The listing builds one solid part. Answer for the finished solid, in the listing's coordinates (mm). Face numbers are marked on the shaded views. A direction names the side the tool comes from. Coordinates: 2 decimals unless noted, no trailing zeros. Order: outer loops, then holes, each group sorted by start corner. A loop starts at its lowest first (then second) coordinate and runs counter-clockwise, first axis right, second up. Notation, with made-up numbers: (23, -27.75) -> (68, -27.75) arc R13 ccw to (68, -5.75) -> close; hole circle Ø7 at (-28.5, -26). An arc over 180 degrees is marked (long way). Write item = value, one per line.
from build123d import *

# Parameters (mm, degrees)
SKETCH_1_W          = 133
SKETCH_1_H          = 140
EXTRUDE_1_DEPTH     = 140
SKETCH_2_W          = 113
SKETCH_2_H          = 100
CUT_EXTRUDE_1_DEPTH = 110
SKETCH_3_W          = 100
SKETCH_3_H          = 13
EXTRUDE_2_DEPTH     = 100
SKETCH_4_R          = 3
CUT_EXTRUDE_3_DEPTH = 217.846143613
SKETCH_5_W          = 12
SKETCH_5_H          = 12
EXTRUDE_3_DEPTH     = 10
SKETCH_6_R          = 14.490887282
SKETCH_6_R_2        = 4.490887282
EXTRUDE_2_2_DEPTH   = 12
SKETCH_7_R          = 4.490887282
CUT_EXTRUDE_4_DEPTH = 265.708919896


with BuildPart() as part:
    # 草圖1 → 填料-伸長1 (new body)
    with BuildSketch(Plane(origin=(0, 0, 0), x_dir=(1, 0, 0), z_dir=(0, 1, 0))):
        Rectangle(SKETCH_1_W, SKETCH_1_H)
    extrude(amount=EXTRUDE_1_DEPTH)

    # 草圖2 → 除料-伸長1 (cut)
    with BuildSketch(Plane(origin=(0, 140, 0), x_dir=(1, 0, 0), z_dir=(0, 1, 0))):
        with Locations((-10, 0)):
            Rectangle(SKETCH_2_W, SKETCH_2_H)
    extrude(amount=-CUT_EXTRUDE_1_DEPTH, mode=Mode.SUBTRACT)

    # 草圖3 → Extrude 2 (add)
    with BuildSketch(Plane.ZY.offset(66.5)):
        with Locations((0, 13.5)):
            Rectangle(SKETCH_3_W, SKETCH_3_H)
    extrude(amount=EXTRUDE_2_DEPTH)

    # 草圖4 → 除料-伸長3 (cut, through all)
    with BuildSketch(Plane(origin=(0, 20, 0), x_dir=(1, 0, 0), z_dir=(0, 1, 0))):
        with Locations(Location((-86.5, 0, 0), (0, 0, 270))):
            Circle(SKETCH_4_R)
    extrude(amount=-CUT_EXTRUDE_3_DEPTH, mode=Mode.SUBTRACT)

    # 草圖5 → 填料-伸長3 (add)
    with BuildSketch(Plane(origin=(0, 0, -70), x_dir=(-1, 0, 0), z_dir=(0, 0, -1))):
        with Locations((-25.5, 126)):
            Rectangle(SKETCH_5_W, SKETCH_5_H)
    extrude(amount=EXTRUDE_3_DEPTH)

    # 草圖6 → Extrude 2 2 (add)
    with BuildSketch(Plane(origin=(31.5, 0, 0), x_dir=(0, 0, -1), z_dir=(1, 0, 0))):
        with Locations((82.5, 132)):
            Circle(SKETCH_6_R)
        with Locations((82.5, 132)):
            Circle(SKETCH_6_R_2, mode=Mode.SUBTRACT)
    extrude(amount=-EXTRUDE_2_2_DEPTH)

    # 草圖7 → 除料-伸長4 (cut, through all)
    with BuildSketch(Plane(origin=(31.5, 0, 0), x_dir=(0, 0, -1), z_dir=(1, 0, 0))):
        with Locations((82.5, 132)):
            Circle(SKETCH_7_R)
    extrude(amount=-CUT_EXTRUDE_4_DEPTH, mode=Mode.SUBTRACT)


solid = part.part
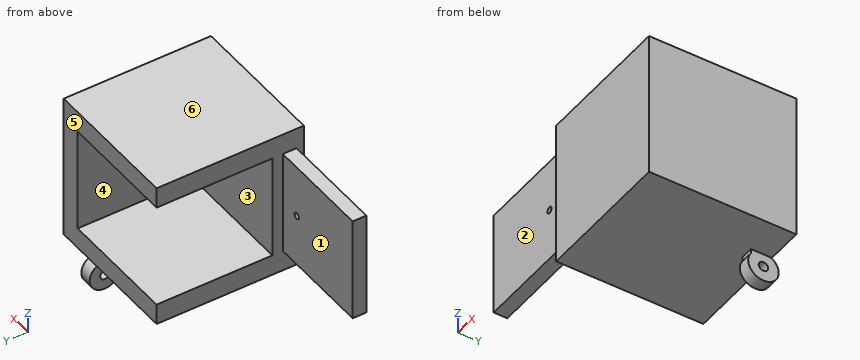
Q1. Section B-B, the plane z = -82.5 is taken. Give the vertices of the cut face in (x, y), plus the area to 3 significant figures.
The answers:
outline = (19.5, 117.51) -> (31.5, 117.51) -> (31.5, 127.51) -> (19.5, 127.51) -> close; (19.5, 136.49) -> (31.5, 136.49) -> (31.5, 146.49) -> (19.5, 146.49) -> close
area = 240 mm2
Q2. The mould has two halves that part along Z. Classify the marked faces 4, 5 and 6: released by +Z, released by -Z, zero draft, split by the parting line, or undercut.
The answers:
face_4 = undercut
face_5 = zero draft
face_6 = released by +Z
Q3. Find the intervals of material crossed by line 1 along X through (y, z) = (15, 0); line 2 along Z through (x, y) = (-38.5, 108); line 3 along Y through (x, z) = (22, -82), in increasing order.
The answers:
line_1 = -166.5 to -89.5, -83.5 to 66.5
line_2 = -70 to -50, 50 to 70
line_3 = 117.52 to 127.54, 136.46 to 146.48
Q4. A tool of negligible diameter and unlimited length cuts with its end or side. For the marked faces 1, 2 and 3, from which of +Z, -Z, +X, -X, +Y, -Y can it reach the whole face along a straight path? Write none if from no direction.
The answers:
face_1 = +Z, -Z, -X, +Y
face_2 = +Z, -Z, -X, -Y
face_3 = -X, +Y
Q5. Section A-A, the plane x = -86.5 is taken. Give the vertices of the cut face in (y, z).
The answers:
outline = (7, -50) -> (20, -50) -> (20, -3) -> (7, -3) -> close; (7, 3) -> (20, 3) -> (20, 50) -> (7, 50) -> close
Q6. Each of these flat-tipped pins is pushed along its axis until it touches: pin 1 Ø8 at (y, z) = (136.5, -87) entering from -X; pin 2 Ø5 at (y, z) = (41.5, 20) entering from -X; pin 3 Ø5 at (x, z) = (-35.5, 13) entering from -Y; pin 4 Ø6.5 at (x, y) = (-102, 10.5) entering from -Z. Where does it stop, or does it pass through?
The answers:
pin_1 = 19.5
pin_2 = 46.5
pin_3 = 0
pin_4 = -50
Q7. Section D-D, the plane x = -21.5 is taken. Give the vertices of the cut face in (y, z), plus the area to 3 significant figures.
The answers:
outline = (0, -70) -> (140, -70) -> (140, -50) -> (30, -50) -> (30, 50) -> (140, 50) -> (140, 70) -> (0, 70) -> close
area = 8,600 mm2
Q8. Section C-C, the plane y = 132 is taken. Give the vertices of the cut face in (x, z).
The answers:
outline = (-66.5, -70) -> (19.5, -70) -> (19.5, -78.01) -> (31.5, -78.01) -> (31.5, -70) -> (66.5, -70) -> (66.5, 70) -> (-66.5, 70) -> (-66.5, 50) -> (46.5, 50) -> (46.5, -50) -> (-66.5, -50) -> close; (19.5, -96.99) -> (31.5, -96.99) -> (31.5, -86.99) -> (19.5, -86.99) -> close
